from build123d import *

# Parameters (mm, degrees)
F0_W     = 60
F0_H     = 60
F1_DEPTH = 5.5
F3_DEPTH = 60
F4_W     = 6.375
F4_H     = 13
F5_DEPTH = 1
F6_W     = 6.375
F6_H     = 45
F6_H_2   = 7
F6_H_3   = 12.4285714286
F6_H_4   = 17.8571428571
F6_H_5   = 23.2857142857
F6_H_6   = 28.7142857143
F6_H_7   = 34.1428571429
F6_H_8   = 39.5714285714
F7_DEPTH = 4.5
F9_DEPTH = 5.5
F9_TAPER = -45


with BuildPart() as f1:
    # F0 (on Top) → F1 (new body)
    with BuildSketch(Plane.XY):
        Rectangle(F0_W, F0_H)
    extrude(amount=F1_DEPTH)

    # F2 (on face) → F3 (cut, through all)
    with BuildSketch(Plane.YZ.offset(30)):
        Polygon((18, 5.5), (30, 2), (30, 5.5), align=None)
    extrude(amount=-F3_DEPTH, mode=Mode.SUBTRACT)

    # F4 (on face) → F5 (cut)
    with BuildSketch(Plane(origin=(0, 0, 0), x_dir=(1, 0, 0), z_dir=(0, 0, -1))):
        with Locations((-25.8125, -23.5)):
            Rectangle(F4_W, F4_H)
        with Locations((-11.0625, -23.5)):
            Rectangle(F4_W, F4_H)
        with Locations((18.4375, -23.5)):
            Rectangle(F4_W, F4_H)
        with Locations((11.0625, -23.5)):
            Rectangle(F4_W, F4_H)
        with Locations((3.6875, -23.5)):
            Rectangle(F4_W, F4_H)
        with Locations((-18.4375, -23.5)):
            Rectangle(F4_W, F4_H)
        with Locations((-3.6875, -23.5)):
            Rectangle(F4_W, F4_H)
        with Locations((25.8125, -23.5)):
            Rectangle(F4_W, F4_H)
    extrude(amount=-F5_DEPTH, mode=Mode.SUBTRACT)

    # F6 (on face) → F7 (cut)
    with BuildSketch(Plane(origin=(0, 0, 0), x_dir=(1, 0, 0), z_dir=(0, 0, -1))):
        with Locations((25.8125, 5.5)):
            Rectangle(F6_W, F6_H)
        with Locations((-25.8125, -13.5)):
            Rectangle(F6_W, F6_H_2)
        with Locations((-18.4375, -10.7857142857)):
            Rectangle(F6_W, F6_H_3)
        with Locations((-11.0625, -8.0714285714)):
            Rectangle(F6_W, F6_H_4)
        with Locations((-3.6875, -5.3571428571)):
            Rectangle(F6_W, F6_H_5)
        with Locations((3.6875, -2.6428571429)):
            Rectangle(F6_W, F6_H_6)
        with Locations((11.0625, 0.0714285714)):
            Rectangle(F6_W, F6_H_7)
        with Locations((18.4375, 2.7857142857)):
            Rectangle(F6_W, F6_H_8)
    extrude(amount=-F7_DEPTH, mode=Mode.SUBTRACT)

    # F8 (on face) → F9 (cut, through all)
    with BuildSketch(Plane(origin=(0, 0, 0), x_dir=(1, 0, 0), z_dir=(0, 0, -1))):
        Polygon((-30, 30), (-30, -3.8595641646), (16, 30), align=None)
    extrude(amount=-F9_DEPTH, taper=F9_TAPER, mode=Mode.SUBTRACT)


solid = f1.part
The listing builds one solid part. Answer for the finished solid, in the listing's coordinates (mm). A direction names the side the tool comes from. Give positions to 0.01 mm unless a question says otherwise; leave off trailing zeros. Answer as a JSON object with one key per item and string values.
1. For faces 1 (the flat face through (-4, -6.286, 2)), 2 (the flat face through (4, 23, 1)), 3 (the flat face through (30, 0, 3)), determine the directions among +Z, -Z, +X, -X, +Y, -Y from which every point of the face is accessible in a straight line to the end or side of a thin tool.
Determined:
{"face 1": "-Z", "face 2": "-Z, +Y", "face 3": "+Z, -Z, +X, +Y, -Y"}
2. Find the intervals of material crossed by L1, parallel to X at y = -18, z = 0.6 (3 decimals); L2, parallel to Y at x = 27.5, z = 1.4; L3, parallel to Z at x = 3, y = -1.5, in increasing order. Write a range as [from, to].
Determined:
{"L1": "[0.71, 15.25], [21.625, 22.625], [29, 30]", "L2": "[-30, -28], [17, 30]", "L3": "[4.5, 5.5]"}
3. A cutting plane is placed at A-A (z = 3.6). Give the number of separate pieces and of enclosed holes in the cut face, then the cut area to 3 significant figures.
Determined:
{"separate pieces": "1", "enclosed holes": "8", "area": "947 mm²"}
4. For a pull along Y with two mould halves and no side action, classify faces 4 (the flat face through (24, -30, 2)), 5 (the flat face through (0, -2, 0)), 6 (the flat face through (-0.5, 8, 2)), 7 (the flat face through (11, -17.143, 2)) as pulls with the +Y half, pulls with the -Y half, needs draft (parallel to the pull), parting line crosses it, or undercut.
Determined:
{"face 4": "pulls with the -Y half", "face 5": "needs draft", "face 6": "undercut", "face 7": "undercut"}
5. Flat-ended cylindrical pins translate along their axes: pin 1 Ø1.9 at (x, y) = (-5.5, 4.5) entering from -Z; pin 2 Ø1.9 at (x, y) = (20, 21) entering from -Z; pin 3 Ø3 at (x, z) = (-6, 2) entering from -Y. Find the tip coordinate at first contact, or state that the pin passes through.
Determined:
{"pin 1": "z = 4.5", "pin 2": "z = 1", "pin 3": "y = -13.49"}
